For this review, take the finished solid that the model builds, in its own axes (mm). A direction names the side the tool comes from. Coordinates: 2 decimals unless noted, no trailing zeros. Write each loop counter-clockwise with the first axis right and the second up, starting at its lowest first coordinate (ties: lowest second). Pieces come first, ordered by that corner, then holes.
1) For faces 1 (the face through (5, -4, -4.5)), 2 (the face through (10, -2, -11)), 3 (the face through (5, 0, -5)), 4 (the face through (5, -10, 0)), 5 (the face through (5, -4.45, -2)), list the 3-axis set-ups (+Z, -Z, +X, -X, +Y, -Y) from which the entire face can be reached by the end or side of a thin tool; tool diameter is ignored.
2) We need section A-A on z = -13.75. Write out the cut boundary in (x, y), then the cut area to 3 significant figures.
3) Mouldability with a two-part tool opening along Y and no side actions: class faces 6 (the face through (0, -2, -11)), 7 (the face through (5, -12, -6)), 8 (the face through (5, -4, -8)) as pulls with the +Y half, pulls with the -Y half, needs draft (parallel to the pull), parting line crosses it, or undercut.
4) We need section C-C on z = -5.75. Write out the cut boundary in (x, y), then the cut area to 3 significant figures.
5) To check wall thickness, follow line 1 along Y through (x, z) = (2.25, -4); line 2 along Y through (x, z) = (3.25, -13.75); line 3 along Z through (x, y) = (3, 1.5). State the ranges of each line that lie inside material, in increasing order.
6) We need section D-D on y = -5. Write out the cut boundary in (x, z), then the cut area to 3 significant figures.
7) We need section B-B on x = 6.25. Write out the cut boundary in (y, z), then the cut area to 3 significant figures.
8) Insertion check: P1, Ø3, axis at x = 2, z = -5, coming from the +Y side; P2, Ø5, axis at y = 2, z = -14, coming from the +X side; P3, Ø2.5, axis at x = 6.5, z = -9, coming from the +Y side; P4, Ø2, axis at y = 2, z = -7, coming from the -X side. Each pin has a flat end and moves straight along its axis. Give the tip position at first contact, or say it passes through.
from build123d import *

# Parameters (mm, degrees)
SKETCH1_R           = 1.45
BOSS_EXTRUDE1_DEPTH = 10
CUT_EXTRUDE1_DEPTH  = 73.480414599
SKETCH3_OUTSIDE_W   = 79.465
SKETCH3_OUTSIDE_H   = 60.027
CUT_EXTRUDE2_DEPTH  = 10


with BuildPart() as part:
    # Sketch1 → Boss-Extrude1 (new body)
    with BuildSketch(Plane(origin=(0, 0, 0), x_dir=(0, 0, -1), z_dir=(1, 0, 0))):
        with BuildLine():
            Line((0, 0), (9.75, 0))
            Line((9.75, 0), (9.75, 3))
            ThreePointArc((9.75, 3), (13.75, 7), (17.75, 3))
            Line((17.75, 3), (17.75, -2.652410493))
            Line((17.75, -2.652410493), (60.297873163, -28.367393861))
            ThreePointArc((60.297873163, -28.367393861), (61.652223967, -33.859727964), (56.159889865, -35.214078769))
            Line((56.159889865, -35.214078769), (17.75, -12))
            Line((17.75, -12), (0, -12))
            Line((0, -12), (0, 0))
        make_face()
        with Locations((13.75, 3)):
            Circle(SKETCH1_R, mode=Mode.SUBTRACT)
        with Locations((58.228881514, -31.790736315)):
            Circle(SKETCH1_R, mode=Mode.SUBTRACT)
    extrude(amount=BOSS_EXTRUDE1_DEPTH)

    # Sketch2 → Cut-Extrude1 (cut, through all)
    with BuildSketch(Plane(origin=(10, 0, 0), x_dir=(0, 0, -1), z_dir=(1, 0, 0))):
        with BuildLine():
            Line((0, -7.55), (0, -4.45))
            Line((0, -4.45), (4.5, -4.45))
            Line((4.5, -4.45), (4.5, -3.65))
            ThreePointArc((4.5, -3.65), (4.646446609, -3.296446609), (5, -3.15))
            Line((5, -3.15), (7.5, -3.15))
            ThreePointArc((7.5, -3.15), (7.853553391, -3.296446609), (8, -3.65))
            Line((8, -3.65), (8, -4.45))
            Line((8, -4.45), (11, -4.45))
            Line((11, -4.45), (11, -7.55))
            Line((11, -7.55), (8, -7.55))
            Line((8, -7.55), (8, -8.35))
            ThreePointArc((8, -8.35), (7.853553391, -8.703553391), (7.5, -8.85))
            Line((7.5, -8.85), (5, -8.85))
            ThreePointArc((5, -8.85), (4.646446609, -8.703553391), (4.5, -8.35))
            Line((4.5, -8.35), (4.5, -7.55))
            Line((4.5, -7.55), (0, -7.55))
        make_face()
    extrude(amount=-CUT_EXTRUDE1_DEPTH, mode=Mode.SUBTRACT)

    # Sketch3 outside → Cut-Extrude2 (cut)
    with BuildSketch(Plane(origin=(10, 0, 0), x_dir=(0, 0, -1), z_dir=(1, 0, 0))):
        with Locations((31.1145, -14.3955)):
            Rectangle(SKETCH3_OUTSIDE_W, SKETCH3_OUTSIDE_H)
        Polygon((17.75, -7), (12.75, -12), (0, -12), (0, 0), (17.75, 43), align=None, mode=Mode.SUBTRACT)
    extrude(amount=-CUT_EXTRUDE2_DEPTH, mode=Mode.SUBTRACT)


solid = part.part
Result:
1. face 1: +X, -X
1. face 2: +Z, -Z, +X, +Y, -Y
1. face 3: +Z, +X, -X, +Y
1. face 4: +Z, +X, -X, +Y, -Y
1. face 5: +Z, +X, -X
2. outline: (0, -11) - (10, -11) - (10, 1.55) - (0, 1.55) - close; (0, 4.45) - (10, 4.45) - (10, 7) - (0, 7) - close
2. area: 151 mm2
3. face 6: needs draft
3. face 7: pulls with the -Y half
3. face 8: undercut
4. outline: (0, -12) - (10, -12) - (10, -8.85) - (0, -8.85) - close; (0, -3.15) - (10, -3.15) - (10, 0) - (0, 0) - close
4. area: 63.0 mm2
5. line 1: y = -12 to -7.55, -4.45 to 0
5. line 2: y = -11 to 1.55, 4.45 to 7
5. line 3: z = -17.75 to -9.75
6. outline: (0, -17.75) - (10, -17.75) - (10, -11) - (0, -11) - close
6. area: 67.5 mm2
7. outline: (-12, -12.75) - (-7, -17.75) - (3, -17.75) arc R4 ccw to (3, -9.75) - (0, -9.75) - (0, 0) - (-4.45, 0) - (-4.45, -4.5) - (-3.65, -4.5) arc R0.5 cw to (-3.15, -5) - (-3.15, -7.5) arc R0.5 cw to (-3.65, -8) - (-4.45, -8) - (-4.45, -11) - (-7.55, -11) - (-7.55, -8) - (-8.35, -8) arc R0.5 cw to (-8.85, -7.5) - (-8.85, -5) arc R0.5 cw to (-8.35, -4.5) - (-7.55, -4.5) - (-7.55, 0) - (-12, 0) - close; hole circle Ø2.9 at (3, -13.75)
7. area: 200 mm2
8. P1: stops at y = 0
8. P2: stops at x = 10
8. P3: stops at y = 4.94
8. P4: passes through
